Check sheet for the modelled part. Datum: model origin and axes. Units: mm. Coordinates: 2 decimals unless noted, no trailing zeros. Loops run counter-clockwise (first coordinate to the right, second up) from the corner with the lowest first, then second, coordinate; pieces in that order, holes last. Notation, with made-up numbers: (-34.5, 6.5) - (-22.5, 6.5) arc R18 cw to (-22.5, 34.5) - close; hole circle Ø7 at (19, 43.5). An arc over 180 degrees is marked (long way). Answer as a JSON object with one key per item and string values. Group by question number.
from build123d import *

# Parameters (mm, degrees)
SKETCH_1_W      = 150
SKETCH_1_H      = 185
SKETCH_1_W_2    = 3.9
SKETCH_1_H_2    = 30.4
SKETCH_1_W_3    = 30.4
SKETCH_1_H_3    = 3.9
EXTRUDE_1_DEPTH = 3.5


with BuildPart() as part:
    # Эскиз1 → Бобышка-Вытянуть1 (new body)
    with BuildSketch(Plane.XY):
        with Locations((75, 92.5)):
            Rectangle(SKETCH_1_W, SKETCH_1_H)
        with Locations((5, 42.5)):
            Rectangle(SKETCH_1_W_2, SKETCH_1_H_2, mode=Mode.SUBTRACT)
        with Locations((5, 142.5)):
            Rectangle(SKETCH_1_W_2, SKETCH_1_H_2, mode=Mode.SUBTRACT)
        with Locations((145, 42.5)):
            Rectangle(SKETCH_1_W_2, SKETCH_1_H_2, mode=Mode.SUBTRACT)
        with Locations((145, 142.5)):
            Rectangle(SKETCH_1_W_2, SKETCH_1_H_2, mode=Mode.SUBTRACT)
        with Locations((75, 5)):
            Rectangle(SKETCH_1_W_3, SKETCH_1_H_3, mode=Mode.SUBTRACT)
        with Locations((75, 180)):
            Rectangle(SKETCH_1_W_3, SKETCH_1_H_3, mode=Mode.SUBTRACT)
    extrude(amount=EXTRUDE_1_DEPTH)


solid = part.part
1. Sectioned sample at B-B on x = 66. Record the cut outline in (y, z).
2. Sectioned sample at C-C on z = 1.4. Record the cut outline in (x, y), plus the area to 3 significant figures.
3. Material ranges on line 1 (X direction, y = 31.5, z = 2.35), recorded low to high.
4. Sectioned sample at A-A on y = 138.5. Record the cut outline in (x, z).
Answers follow:
{
 "1": {"outline": "(0, 0) - (3.05, 0) - (3.05, 3.5) - (0, 3.5) - close; (6.95, 0) - (178.05, 0) - (178.05, 3.5) - (6.95, 3.5) - close; (181.95, 0) - (185, 0) - (185, 3.5) - (181.95, 3.5) - close"},
 "2": {"outline": "(0, 0) - (150, 0) - (150, 185) - (0, 185) - close; hole (3.05, 27.3) - (6.95, 27.3) - (6.95, 57.7) - (3.05, 57.7) - close; hole (3.05, 127.3) - (6.95, 127.3) - (6.95, 157.7) - (3.05, 157.7) - close; hole (59.8, 3.05) - (90.2, 3.05) - (90.2, 6.95) - (59.8, 6.95) - close; hole (59.8, 178.05) - (90.2, 178.05) - (90.2, 181.95) - (59.8, 181.95) - close; hole (143.05, 27.3) - (146.95, 27.3) - (146.95, 57.7) - (143.05, 57.7) - close; hole (143.05, 127.3) - (146.95, 127.3) - (146.95, 157.7) - (143.05, 157.7) - close", "area": "27,000 mm^2"},
 "3": {"line 1": "x = 0 to 3.05, 6.95 to 143.05, 146.95 to 150"},
 "4": {"outline": "(0, 0) - (3.05, 0) - (3.05, 3.5) - (0, 3.5) - close; (6.95, 0) - (143.05, 0) - (143.05, 3.5) - (6.95, 3.5) - close; (146.95, 0) - (150, 0) - (150, 3.5) - (146.95, 3.5) - close"}
}
